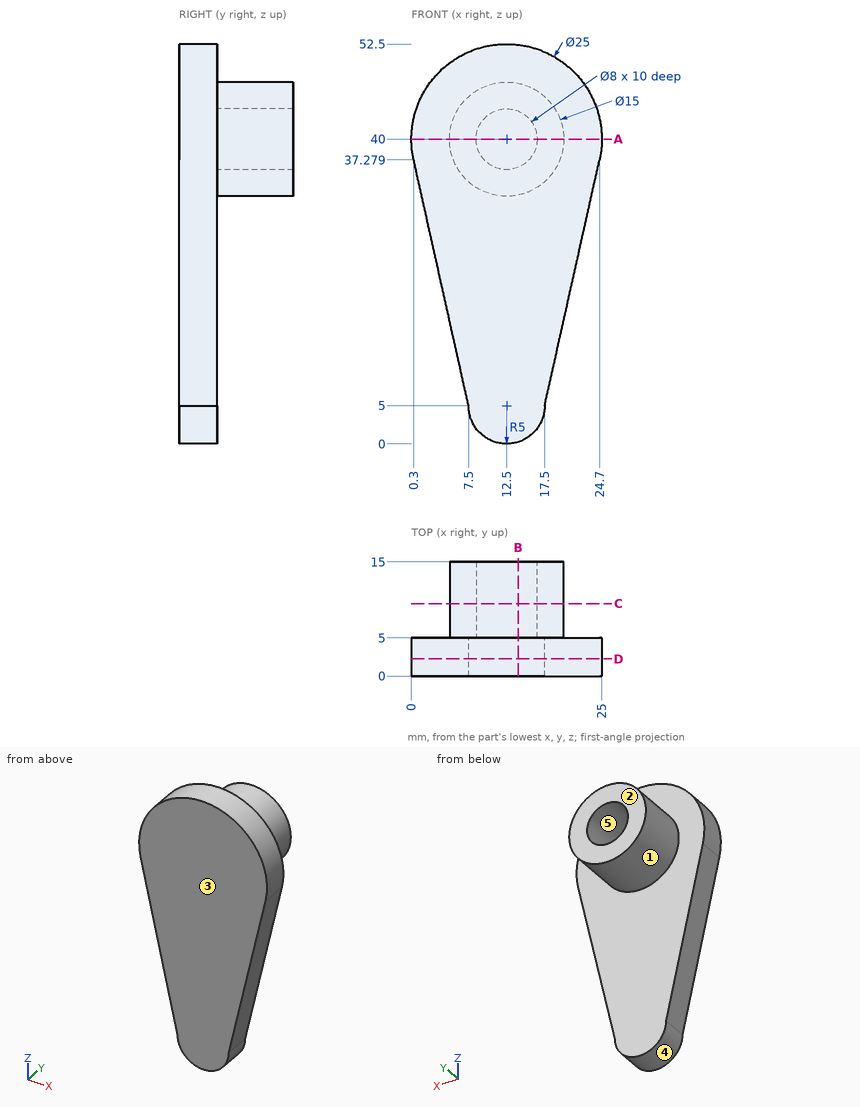
Drawing for the job (mm, zero at the part's lowest x, y, z). A direction names the side the tool comes from. Give positions to 0.01 mm unless a question says otherwise; leave off trailing zeros. Order: outer loops, then holes, each group sorted by start corner. A loop starts at its lowest first (then second) coordinate and runs counter-clockwise, first axis right, second up. Notation, with made-up numbers: M 16.25,21.5 L 40.25,21.5 A20 ccw 40.25,60.5 Z; hole C 24.25,-2 d4. An arc over 180 degrees is marked long. Put each result on its own line as item: value. Start each with the question number.
(1) Saw through at A-A, the plane z = 40. Write the cut outline in (x, y).
(2) Flat gauge pins, fed straight in: pin 1 Ø1.5 at (x, y) = (18.5, 13.5) entering from +Z (1 decimal); pin 2 Ø6.5 at (x, z) = (12.5, 40.5) entering from +Y; pin 3 Ø4 at (x, y) = (16.5, 3) entering from -Z; pin 4 Ø1.5 at (x, y) = (22.5, 10.5) entering from +Z. Where does each tip first touch, or does it go through?
(3) Saw through at D-D, the plane y = 2.25. Write the cut outline in (x, z).
(4) Which spindle directions (+Z, -Z, +X, -X, +Y, -Y) get a long thin tool onto all of the face, cutting with end or side? Do the marked faces 1 and 2. Say none if no direction does.
(5) Drill centre lines: line 1 along X through (y, z) = (9, 40); line 2 along Y through (x, z) = (15, 48.5); line 3 along X through (y, z) = (9, 38) (1 decimal). Where is each one in solid material? Low to high.
(6) Mould opens along X. For the marked faces 3, 4 and 5 say: +X half, -X half, draft (parallel to the pull), parting line (faces both ways), or undercut.
(7) Saw through at C-C, the plane y = 9.5. Write the cut outline in (x, z).
(8) Saw through at B-B, the plane x = 14. Write the cut outline in (y, z).
Check result:
1. outline: M 0,0 L 25,0 L 25,5 L 20,5 L 20,15 L 16.5,15 L 16.5,5 L 8.5,5 L 8.5,15 L 5,15 L 5,5 L 0,5 Z
2. pin 1: stops at z = 45.4
2. pin 2: stops at y = 5
2. pin 3: stops at z = 0.42
2. pin 4: passes through
3. outline: M 0.3,37.28 L 7.5,5 A5 ccw 17.5,5 L 24.7,37.28 A12.5 ccw long Z
4. face 1: +Y
4. face 2: +Z, -Z, +X, -X, +Y
5. line 1: x = 5 to 8.5, 16.5 to 20
5. line 2: y = 0 to 5
5. line 3: x = 5.3 to 9, 16 to 19.7
6. face 3: draft
6. face 4: parting line
6. face 5: undercut
7. outline: C 12.5,40 d15; hole C 12.5,40 d8
8. outline: M 0,0.23 L 5,0.23 L 5,32.65 L 15,32.65 L 15,36.29 L 5,36.29 L 5,43.71 L 15,43.71 L 15,47.35 L 5,47.35 L 5,52.41 L 0,52.41 Z
